For this review, take the finished solid that the model builds, in its own axes (mm). Give positions to 0.01 mm unless a question says otherwise; leave off trailing zeros. Write each loop counter-clockwise with the first axis right and the second up, starting at its lowest first coordinate (ties: lowest second). Pieces come first, ordered by that corner, then holes.
1) We need section A-A on z = 8.5. Give the boundary of the cut face in (x, y), and give its area (3 significant figures).
2) We need section B-B on y = 34. Give the boundary of the cut face in (x, z).
3) Wall thickness on line 1 along Y through (x, z) = (8.5, 59); line 2 along Z through (x, y) = (14.5, 1); line 3 along Y through (x, z) = (15, 72.5): over which ranges is each line inside the solid? List them lowest first.
4) For P1, Ø6, axis at x = -2, z = 35, coming from the +Y side; P2, Ø5.5, axis at x = -22, y = -12.5, coming from the -Z side; P3, Ø12, axis at x = -4.5, z = 28, coming from the +Y side; P4, Ø5, axis at x = 10, y = 19.5, coming from the -Z side, all flat-tipped, find the tip position at first contact; note any pin that passes through.
from build123d import *

# Parameters (mm, degrees)
SKETCH_1_W      = 17
SKETCH_1_H      = 40
EXTRUDE_1_DEPTH = 10
SKETCH_2_W      = 17
SKETCH_2_H      = 40
EXTRUDE_2_DEPTH = 20
EXTRUDE_2_TAPER = -30
EXTRUDE_3_DEPTH = 25


with BuildPart() as part:
    # 草图1 → 凸台-拉伸1 (new body)
    with BuildSketch(Plane.XY):
        Rectangle(SKETCH_1_W, SKETCH_1_H)
    extrude(amount=EXTRUDE_1_DEPTH)

    # 草图2 → 凸台-拉伸2 (add)
    with BuildSketch(Plane.XY.offset(10)):
        Rectangle(SKETCH_2_W, SKETCH_2_H)
    extrude(amount=EXTRUDE_2_DEPTH, taper=EXTRUDE_2_TAPER)

    # 草图3 → 凸台-拉伸3 (add, symmetric)
    with BuildSketch(Plane(origin=(0, 0, 0), x_dir=(0, 0, -1), z_dir=(1, 0, 0))):
        with BuildLine():
            Line((-30, 31.547005384), (-30, -31.547005384))
            ThreePointArc((-30, -31.547005384), (-116.885818272, 0), (-30, 31.547005384))
        make_face()
    extrude(amount=EXTRUDE_3_DEPTH, both=True)


solid = part.part
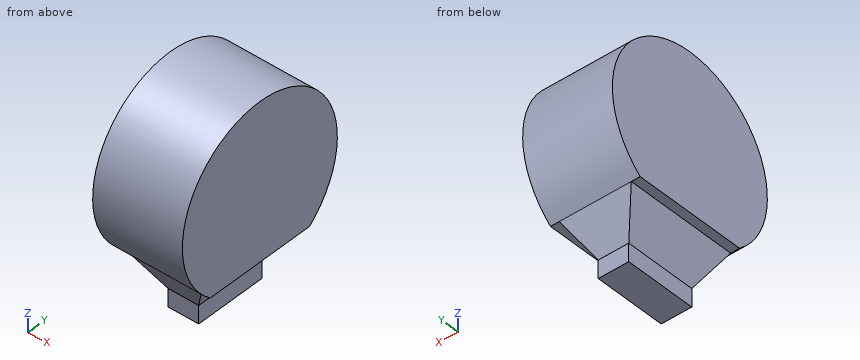
Results list:
1. outline: (-8.5, -20) - (8.5, -20) - (8.5, 20) - (-8.5, 20) - close
1. area: 680 mm2
2. outline: (-25, 32.2) - (25, 32.2) - (25, 103.24) - (-25, 103.24) - close
3. line 1: y = -48.39 to 48.39
3. line 2: z = 20.39 to 116.88
3. line 3: y = -48.94 to 48.94
4. P1: stops at y = 39.17
4. P2: stops at z = 28.62
4. P3: stops at y = 35.79
4. P4: stops at z = 0
